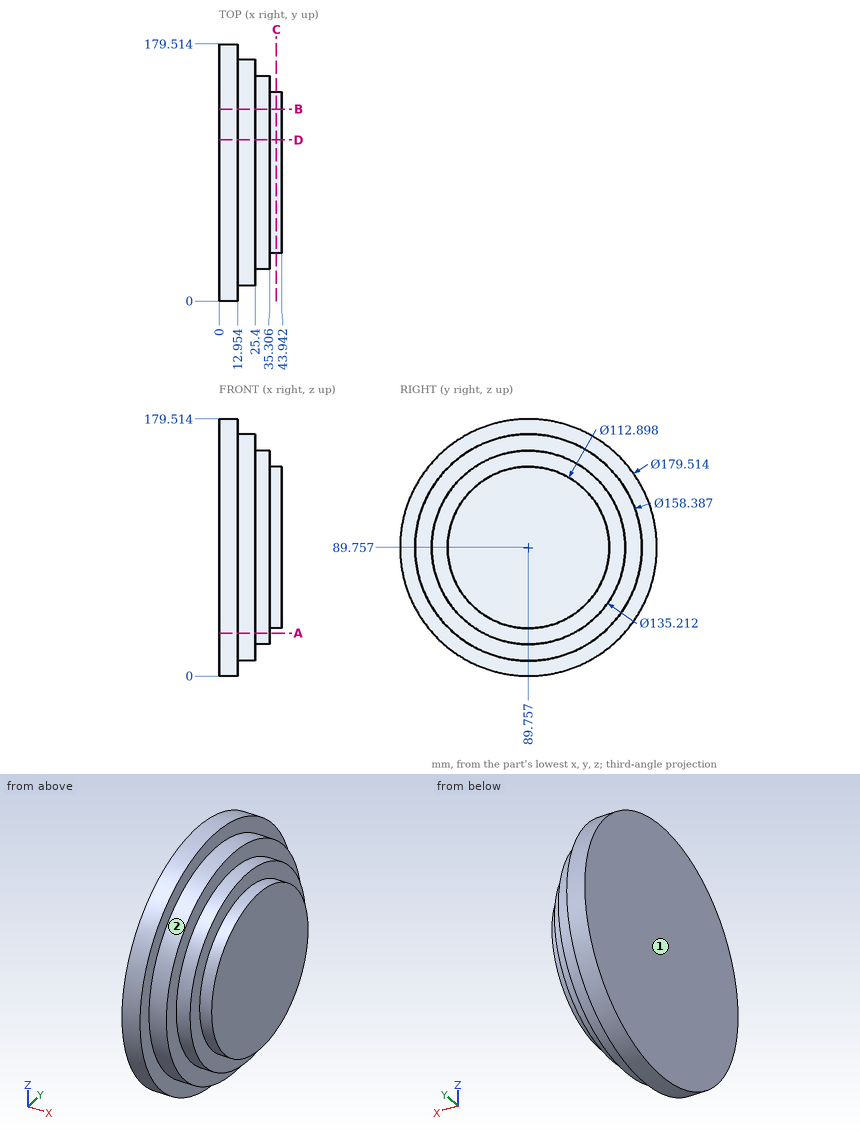
Design review of the part shown in the three views and the two pictorial views. Dimensions are in mm from the part's minimum x, y and z. A direction names the side the tool comes from. Round coordinates to 2 decimals unless told otherwise and drop trailing zeros. Order: outer loops, then holes, each group sorted by start corner. A loop starts at its lowest first (then second) coordinate and runs counter-clockwise, first axis right, second up.
(1) Wall thickness on L1, parallel to X at y = 129, z = 38.5; L2, parallel to Y at x = 30, z = 91.5; L3, parallel to X at y = 165, z = 70: over which ranges is each line inside the solid? List them lowest first.
Working result:
L1: x = 0 to 35.31
L2: y = 22.17 to 157.34
L3: x = 0 to 25.4
(2) Take a section at B-B, the plane y = 134. State the section outline as (x, z) points (1 decimal).
Working result:
outline: (0, 11.7) - (13, 11.7) - (13, 24.1) - (25.4, 24.1) - (25.4, 38.6) - (35.3, 38.6) - (35.3, 54.7) - (43.9, 54.7) - (43.9, 124.8) - (35.3, 124.8) - (35.3, 140.9) - (25.4, 140.9) - (25.4, 155.4) - (13, 155.4) - (13, 167.9) - (0, 167.9) - close
(3) Take a section at A-A, the plane z = 30. State the section outline as (x, y) points (1 decimal), plus the area to 4 significant figures.
Working result:
outline: (0, 22.8) - (13, 22.8) - (13, 37.8) - (25.4, 37.8) - (25.4, 58.1) - (35.3, 58.1) - (35.3, 121.4) - (25.4, 121.4) - (25.4, 141.7) - (13, 141.7) - (13, 156.7) - (0, 156.7) - close
area: 3,655 mm2
(4) Tool access review of the marked faces 1 and 2: name each direction out of +Z, -Z, +X, -X, +Y, -Y from which nothing blocks a thin tool from reaching the whole face with its end or side.
Working result:
face 1: +Z, -Z, -X, +Y, -Y
face 2: +X
(5) Take a section at D-D, the plane y = 112.5. State the section outline as (x, z) points (1 decimal).
Working result:
outline: (0, 2.9) - (13, 2.9) - (13, 13.9) - (25.4, 13.9) - (25.4, 26.1) - (35.3, 26.1) - (35.3, 38.1) - (43.9, 38.1) - (43.9, 141.4) - (35.3, 141.4) - (35.3, 153.4) - (25.4, 153.4) - (25.4, 165.6) - (13, 165.6) - (13, 176.6) - (0, 176.6) - close
(6) For P1, Ø2, axis at x = 18.5, y = 158.5, coming from the +Z side (1 decimal); P2, Ø5, axis at x = 22.5, y = 138.5, coming from the -Z side; P3, Ø12, axis at x = 29.5, z = 98, coming from the +Y side, all flat-tipped, find the tip position at first contact; note any pin that passes through.
Working result:
P1: stops at z = 130.8
P2: stops at z = 25.47
P3: stops at y = 168.86
(7) Take a section at C-C, the plane x = 40. State the section outline as (y, z) points.
Working result:
outline: circle Ø112.9 at (89.76, 89.76)
